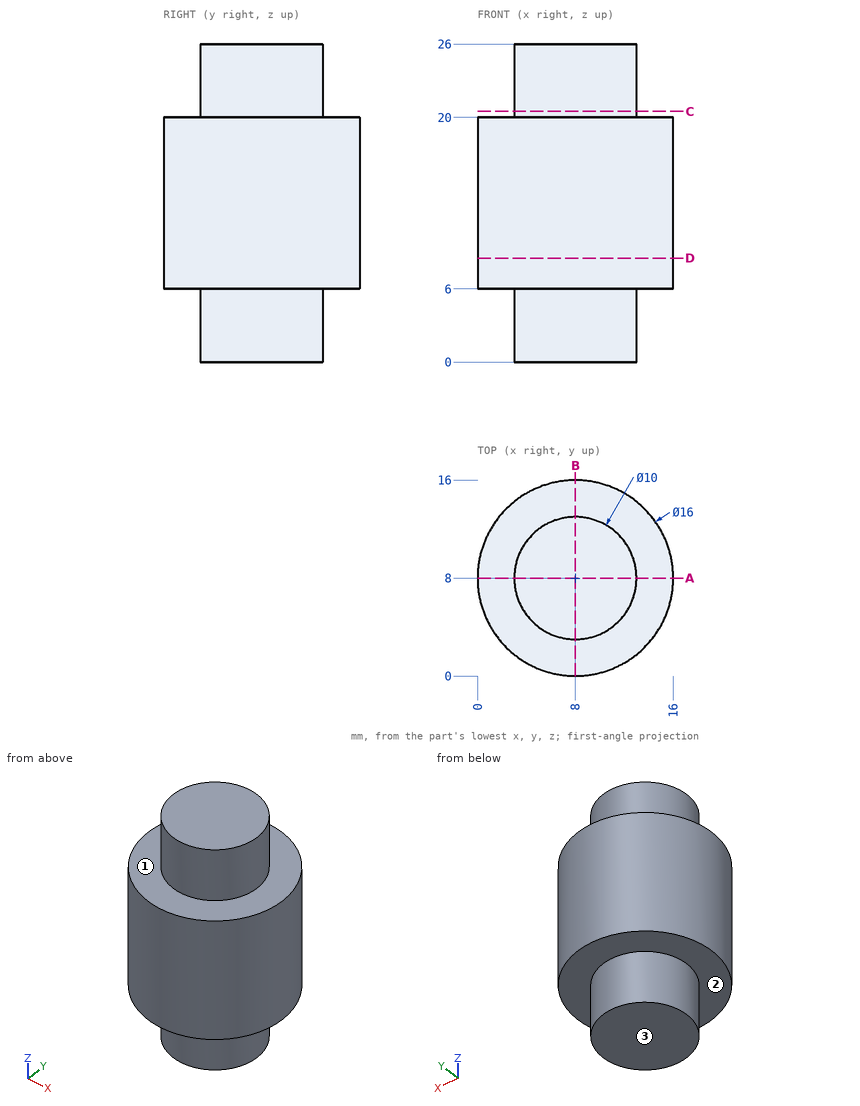
Drawing for the job (mm, zero at the part's lowest x, y, z). A direction names the side the tool comes from. Round coordinates to 2 decimals unless told otherwise and drop trailing zeros. Write each loop counter-clockwise with the first axis right and the second up, starting at its lowest first coordinate (ties: lowest second). Pieces come first, ordered by that corner, then holes. Notation, with made-up numbers: M -32,84 L 15,84 A11 cw 15,104 Z; hole C 12,33.25 d9. An arc over 180 degrees is marked long. Answer as a JSON object with one key per item and string values. Group by question number.
(1) Cut at D-D (z = 8.5). Give the cut face in (x, y).
(2) Cut at C-C (z = 20.5). Give the cut face in (x, y), and give its area (3 significant figures).
(3) Flat gauge pins, fed straight in: pin 1 (8 mm diameter, centred on x = 13.5, z = 22, fed in from -Y); pin 2 (1 mm diameter, centred on y = 10.5, z = 19.5, fed in from -X); pin 3 (6 mm diameter, centred on y = 13.5, z = 20, fed in from +X); pin 4 (4 mm diameter, centred on y = 9, z = 6, fed in from -X). Where does each tip first touch, or does it go through?
(4) Drill centre lines: L1, parallel to Z at x = 2.5, y = 3; L2, parallel to Y at x = 4.5, z = 6.75; L3, parallel to X at y = 7, z = 18.25. Where is each one in solid material? Low to high.
(5) Cut at A-A (y = 8). Give the cut face in (x, z).
(6) Which spindle directions (+Z, -Z, +X, -X, +Y, -Y) get a long thin tool onto all of the face, cutting with end or side? Do the marked faces 1, 2 and 3. Say none if no direction does.
Responses:
{
 "1": {"outline": "C 8,8 d16"},
 "2": {"outline": "C 8,8 d10", "area": "78.5 mm2"},
 "3": {"pin 1": "stops at y = 0.26", "pin 2": "stops at x = 0.25", "pin 3": "stops at x = 15.6", "pin 4": "stops at x = 0"},
 "4": {"L1": "z = 6 to 20", "L2": "y = 0.81 to 15.19", "L3": "x = 0.06 to 15.94"},
 "5": {"outline": "M 0,6 L 3,6 L 3,0 L 13,0 L 13,6 L 16,6 L 16,20 L 13,20 L 13,26 L 3,26 L 3,20 L 0,20 Z"},
 "6": {"face 1": "+Z", "face 2": "-Z", "face 3": "-Z, +X, -X, +Y, -Y"}
}
